The figure shows three views and two pictorial views of one solid part (mm, origin at its lowest corner). Answer the questions. A direction names the side the tool comes from. Coordinates: 2 decimals unless noted, no trailing zeros. Loops run counter-clockwise (first coordinate to the right, second up) from the corner with the lowest first, then second, coordinate; pieces in that order, holes last. Notation, with made-up numbers: M -23,11.5 L -6,11.5 A15 cw -6,16.5 Z; hole C 45.5,54.25 d1. An arc over 180 degrees is marked long. Return JSON: item names as keys, results as strings. Group by question number.
1. Given P1, Ø6, axis at y = 34.5, z = 7, coming from the -X side; P2, Ø12, axis at y = 9, z = 8.5, coming from the -X side (1 decimal); P3, Ø4, axis at y = 9, z = 21.5, coming from the -X side (1 decimal), each flat-ended and moving along its own axis, determine where each tip first touches the part or whether it passes through.
2. Section D-D (x = 31) is taken. Write down the section's boundary in (y, z) (1 decimal), then the cut area to 3 significant figures.
3. Section C-C (x = 21) is taken. Write down the section's boundary in (y, z) (1 decimal).
4. Which of the six approach directions +Z, -Z, +X, -X, +Y, -Y give full straight-line access (tool end or side, diameter ignored) to the marked faces 1 and 2?
5. Straight lines are drawn through the part: L1, parallel to X at y = 41, z = 18 (1 decimal); L2, parallel to Z at x = 11, y = 17 (1 decimal); L3, parallel to X at y = 25, z = 1. For each, find the intervals that lie inside material, in ascending order. Write a range as from..to.
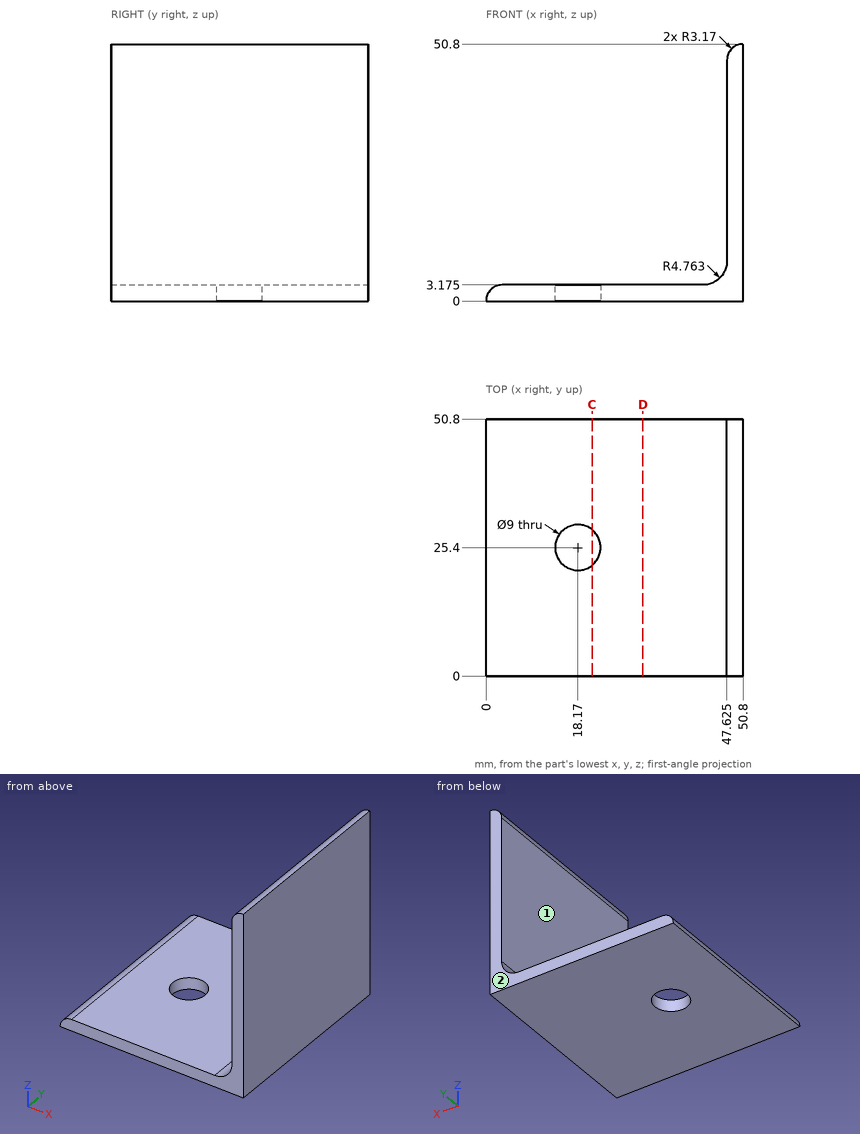
Worked out:
{
 "1": {"P1": "x = 45.54", "P2": "x = 1.2", "P3": "x = 47.6"},
 "2": {"outline": "M 0,0 L 50.8,0 L 50.8,3.2 L 0,3.2 Z", "area": "161 mm^2"},
 "3": {"outline": "M 0,0 L 21.9,0 L 21.9,3.2 L 0,3.2 Z; M 28.9,0 L 50.8,0 L 50.8,3.2 L 28.9,3.2 Z"},
 "4": {"face 1": "+Z, -X, +Y, -Y", "face 2": "+Z, -Z, +X, -X, +Y"},
 "5": {"L1": "47.6..50.8", "L2": "0..3.2", "L3": "0.16..13.69, 22.65..50.8"}
}
